from build123d import *

# Parameters (mm, degrees)
EXTRUDE1_REACH            = 119.713
SKETCH2_W                 = 8
SKETCH2_H                 = 10
SKETCH3_W                 = 13.5
SKETCH3_H                 = 4
SKETCH5_W                 = 15.5
SKETCH5_H                 = 4.8
EXTRUDE3_DEPTH            = 40
SKETCH6_R                 = 1.65
EXTRUDE4_DEPTH            = 10
M8X1_0_TAPPED_HOLE1_D     = 7
M8X1_0_TAPPED_HOLE1_DEPTH = 20
M8X1_0_TAPPED_HOLE1_TIP   = 2.103012167
M6X1_0_TAPPED_HOLE1_D     = 5
M6X1_0_TAPPED_HOLE1_DEPTH = 26.5


with BuildPart() as part:
    # Sketch1 → Revolve1 (revolve)
    with BuildSketch(Plane.XY, mode=Mode.PRIVATE) as revolve1_sk:
        Polygon((-6.5, 26.3), (-19, 26.3), (-19, 106.8), (-35, 106.8), (-35, 19), (-19, 19), (-19, 0), (-10, 0), (-10, 15), (-6.5, 15), align=None)
    revolve(revolve1_sk.sketch.rotate(Axis((0, 0, 0), (0, 1, 0)), 270), axis=Axis((0, 0, 0), (0, 1, 0)))

    # Sketch2 → Extrude1 (cut, up to next)
    with BuildSketch(Plane(origin=(0, 106.8, 0), x_dir=(1, 0, 0), z_dir=(0, 1, 0)), mode=Mode.PRIVATE) as extrude1_sk1:
        with Locations((-18, 0)):
            Rectangle(SKETCH2_W, SKETCH2_H)
    extrude1_tool1 = extrude(extrude1_sk1.sketch, amount=-EXTRUDE1_REACH, mode=Mode.PRIVATE) & part.part
    add(extrude1_tool1.solids().sort_by_distance((-18, 106.8, 0))[0], mode=Mode.SUBTRACT)

    # Sketch3 → Revolve2 (revolve)
    with BuildSketch(Plane.XY, mode=Mode.PRIVATE) as revolve2_sk:
        with Locations((-41.75, 80.8)):
            Rectangle(SKETCH3_W, SKETCH3_H)
    revolve(revolve2_sk.sketch.rotate(Axis((0, 0, 0), (0, 1, 0)), 270), axis=Axis((0, 0, 0), (0, 1, 0)))

    # Sketch5 → Extrude3 (cut, symmetric)
    with BuildSketch(Plane(origin=(0, 0, 0), x_dir=(0, 0, -1), z_dir=(1, 0, 0))):
        with Locations((28.25, 21.4)):
            Rectangle(SKETCH5_W, SKETCH5_H)
        with Locations((-28.25, 21.4)):
            Rectangle(SKETCH5_W, SKETCH5_H)
    extrude(amount=EXTRUDE3_DEPTH, both=True, mode=Mode.SUBTRACT)

    # Sketch6 → Extrude4 (cut)
    with BuildSketch(Plane(origin=(0, 82.8, 0), x_dir=(1, 0, 0), z_dir=(0, 1, 0))):
        with Locations(Location((0, -44, 0), (0, 0, 270))):
            Circle(SKETCH6_R)
        with Locations(Location((-38.105117767, -22, 0), (0, 0, 270))):
            Circle(SKETCH6_R)
        with Locations(Location((-38.105117767, 22, 0), (0, 0, 270))):
            Circle(SKETCH6_R)
        with Locations(Location((0, 44, 0), (0, 0, 270))):
            Circle(SKETCH6_R)
        with Locations(Location((38.105117767, 22, 0), (0, 0, 270))):
            Circle(SKETCH6_R)
        with Locations(Location((38.105117767, -22, 0), (0, 0, 270))):
            Circle(SKETCH6_R)
    extrude(amount=-EXTRUDE4_DEPTH, mode=Mode.SUBTRACT)

    # M8x1.0 Tapped Hole1
    with Locations(Plane(origin=(-35, 19, 0), x_dir=(-1, 0, 0), z_dir=(0, -1, 0))):
        with Locations((-62.5, 0), (-7.5, 0), (-35, 27.5), (-35, -27.5)):
            Hole(M8X1_0_TAPPED_HOLE1_D / 2, depth=M8X1_0_TAPPED_HOLE1_DEPTH)
            with Locations((0, 0, -(M8X1_0_TAPPED_HOLE1_DEPTH + M8X1_0_TAPPED_HOLE1_TIP / 2))):  # 118° drill point
                Cone(0, M8X1_0_TAPPED_HOLE1_D / 2, M8X1_0_TAPPED_HOLE1_TIP, mode=Mode.SUBTRACT)

    # M6x1.0 Tapped Hole1
    with Locations(Plane(origin=(-22, 0, 0), x_dir=(0, 0, -1), z_dir=(1, 0, 0))):
        with Locations((0, 56.8)):
            Hole(M6X1_0_TAPPED_HOLE1_D / 2, depth=M6X1_0_TAPPED_HOLE1_DEPTH)


solid = part.part
The model under review builds one solid part; all positions refer to its coordinate system, in mm. A direction names the side the tool comes from. Give positions to 0.01 mm unless a question says otherwise; leave off trailing zeros. Write each loop counter-clockwise with the first axis right and the second up, starting at its lowest first coordinate (ties: lowest second). Pieces come first, ordered by that corner, then holes.
1. Tool access review of faces 4 (the flat face through (0, 23.8, -23)), 5 (the cylindrical face through (21, 95, 28)), 6 (the flat face through (0, 21, 20.5)): name each direction out of +Z, -Z, +X, -X, +Y, -Y from which nothing blocks a thin tool from reaching the whole face with its end or side.
2. Draft analysis for pull direction Y (two halves, no side actions). For faces 1 (the cylindrical face through (-28.59, 59.28, -0.33)), 2 (the flat face through (0, 23.8, 23)), 3 (the cylindrical face through (30.84, 29.14, -1.05)), state which applies: +Y half, -Y half, draft (parallel to the pull), parting line (faces both ways), or undercut.
3. Wall thickness on L1, parallel to X at y = 63, z = 0; L2, parallel to X at y = 80.8, z = -22; L3, parallel to Y at x = -23, z = 21: over which ranges is each line inside the solid? List them lowest first.
4. For P1, Ø16, axis at x = 14, z = -28, coming from the -Y side; P2, Ø2.5, axis at x = -17.5, y = 50, coming from the -Z side; P3, Ø7.5, axis at x = 13.5, z = 31, coming from the -Y side, all flat-tipped, find the tip position at first contact; note any pin that passes through.
5. Add section B-B, the plane z = -22. Write out the cut boundary in (x, y), plus the area to 3 significant figures.
6. Add section A-A, the plane y = 21.5. Write out the cut boundary in (x, z).
7. Add section D-D, the plane z = -44. Write out the cut boundary in (x, y).
8. Add section C-C, the plane y = 98.5. Write out the cut boundary in (x, z), plus the area to 3 significant figures.
Worked answers:
1. face 4: -Z, +X, -X, -Y
1. face 5: +Y
1. face 6: +Z, +X, -X, -Y
2. face 1: undercut
2. face 2: -Y half
2. face 3: draft
3. L1: x = -35 to -22, 19 to 35
3. L2: x = -43.22 to -39.76, -36.46 to 36.46, 39.76 to 43.22
3. L3: y = 23.8 to 106.8
4. P1: stops at y = 19
4. P2: stops at z = -31
4. P3: stops at y = 23.8
5. outline: (-43.22, 78.8) - (-39.76, 78.8) - (-39.76, 82.8) - (-43.22, 82.8) - close; (-36.46, 78.8) - (-27.22, 78.8) - (-27.22, 23.8) - (27.22, 23.8) - (27.22, 78.8) - (36.46, 78.8) - (36.46, 82.8) - (27.22, 82.8) - (27.22, 106.8) - (-27.22, 106.8) - (-27.22, 82.8) - (-36.46, 82.8) - close; (39.76, 78.8) - (43.22, 78.8) - (43.22, 82.8) - (39.76, 82.8) - close
5. area: 4,620 mm2
6. outline: (-28.37, -20.5) - (28.37, -20.5) arc R35 ccw to (28.37, 20.5) - (-28.37, 20.5) arc R35 ccw to start; hole circle Ø7 at (-27.5, 0); hole (-22, -5) - (-14, -5) - (-14, 5) - (-22, 5) - close; hole circle Ø13 at (0, 0); hole circle Ø7 at (27.5, 0)
7. outline: (-20.4, 78.8) - (-1.65, 78.8) - (-1.65, 82.8) - (-20.4, 82.8) - close; (1.65, 78.8) - (20.4, 78.8) - (20.4, 82.8) - (1.65, 82.8) - close
8. outline: circle Ø70 at (0, 0); hole (-22, -5) - (-18.33, -5) arc R19 ccw (long way) to (-18.33, 5) - (-22, 5) - close
8. area: 2,680 mm2
